```python
from build123d import *

# Parameters (mm, degrees)
SKETCH1_R               = 17.78
BOSS_EXTRUDE1_DEPTH     = 177.8
SKETCH9_R               = 23.495
BOSS_EXTRUDE4_DEPTH     = 12.7
MIRROR6_COPY_1_SKETCH_R = 23.495
MIRROR6_COPY_1_DEPTH    = 12.7
MIRROR6_COPY_2_SKETCH_R = 23.495
MIRROR6_COPY_2_DEPTH    = 12.7
MIRROR7_COPY_1_SKETCH_R = 23.495
MIRROR7_COPY_1_DEPTH    = 12.7
MIRROR7_COPY_2_SKETCH_R = 23.495
MIRROR7_COPY_2_DEPTH    = 12.7
MIRROR7_COPY_3_SKETCH_R = 23.495
MIRROR7_COPY_3_DEPTH    = 12.7
SKETCH13_R              = 88.9
BOSS_EXTRUDE6_DEPTH     = 76.2
FILLET3_R               = 25.4
FILLET4_R               = 25.4
FILLET3_OF_MIRROR11_R   = 25.4
FILLET4_OF_MIRROR11_R   = 25.4


with BuildPart() as part:
    # Sketch1 → Boss-Extrude1 (new, symmetric)
    with BuildSketch(Plane(origin=(0, 0, 0), x_dir=(0, 0, -1), z_dir=(1, 0, 0))):
        Circle(SKETCH1_R)
    extrude(amount=BOSS_EXTRUDE1_DEPTH, both=True)

    # Sketch9 → Boss-Extrude4 (add)
    with BuildSketch(Plane(origin=(177.8, 0, 0), x_dir=(0, 0, -1), z_dir=(1, 0, 0))):
        Circle(SKETCH9_R)
    boss_extrude4 = extrude(amount=BOSS_EXTRUDE4_DEPTH)

    # Mirror5: Boss-Extrude4 across plane
    add(boss_extrude4.mirror(Plane(origin=(0, 0, 0), x_dir=(0, 0, 1), z_dir=(1, 0, 0))))

    # Mirror6 copy 1 sketch → Mirror6 copy 1 (add)
    with BuildSketch(Plane.ZY.offset(177.8)):
        Circle(MIRROR6_COPY_1_SKETCH_R)
    extrude(amount=MIRROR6_COPY_1_DEPTH)

    # Mirror6 copy 2 sketch → Mirror6 copy 2 (add)
    with BuildSketch(Plane(origin=(177.8, 0, 0), x_dir=(0, 0, 1), z_dir=(1, 0, 0))):
        Circle(MIRROR6_COPY_2_SKETCH_R)
    extrude(amount=MIRROR6_COPY_2_DEPTH)

    # Mirror7 copy 1 sketch → Mirror7 copy 1 (add)
    with BuildSketch(Plane(origin=(-177.8, 0, 0), x_dir=(0, 0, -1), z_dir=(-1, 0, 0))):
        Circle(MIRROR7_COPY_1_SKETCH_R)
    extrude(amount=MIRROR7_COPY_1_DEPTH)

    # Mirror7 copy 2 sketch → Mirror7 copy 2 (add)
    with BuildSketch(Plane(origin=(177.8, 0, 0), x_dir=(0, 0, -1), z_dir=(1, 0, 0))):
        Circle(MIRROR7_COPY_2_SKETCH_R)
    extrude(amount=MIRROR7_COPY_2_DEPTH)

    # Mirror7 copy 3 sketch → Mirror7 copy 3 (add)
    with BuildSketch(Plane(origin=(177.8, 0, 0), x_dir=(0, 0, 1), z_dir=(1, 0, 0))):
        Circle(MIRROR7_COPY_3_SKETCH_R)
    extrude(amount=MIRROR7_COPY_3_DEPTH)

    # Sketch13 → Boss-Extrude6 (add)
    with BuildSketch(Plane(origin=(190.5, 0, 0), x_dir=(0, 0, -1), z_dir=(1, 0, 0))):
        with Locations(Location((0, 0, 0), (0, 0, 180))):
            Circle(SKETCH13_R)
    boss_extrude6 = extrude(amount=BOSS_EXTRUDE6_DEPTH)

    # Fillet3
    fillet3_edges = [part.edges().sort_by_distance(p)[0] for p in [
        (266.7, 0, -88.9),
    ]]
    fillet(fillet3_edges, radius=FILLET3_R)

    # Fillet4
    fillet4_edges = [part.edges().sort_by_distance(p)[0] for p in [
        (190.5, 0, -88.9),
    ]]
    fillet(fillet4_edges, radius=FILLET4_R)

    # Mirror11: Boss-Extrude6 across plane
    add(boss_extrude6.mirror(Plane(origin=(0, 0, 0), x_dir=(0, 0, 1), z_dir=(1, 0, 0))))

    # Fillet3 of Mirror11
    fillet3_of_mirror11_edges = [part.edges().sort_by_distance(p)[0] for p in [
        (-266.7, 0, -88.9),
    ]]
    fillet(fillet3_of_mirror11_edges, radius=FILLET3_OF_MIRROR11_R)

    # Fillet4 of Mirror11
    fillet4_of_mirror11_edges = [part.edges().sort_by_distance(p)[0] for p in [
        (-190.5, 0, -88.9),
    ]]
    fillet(fillet4_of_mirror11_edges, radius=FILLET4_OF_MIRROR11_R)


solid = part.part
```
The listing builds one solid part. Answer for the finished solid, in the listing's coordinates (mm). A direction names the side the tool comes from. Round coordinates to 2 decimals unless told otherwise and drop trailing zeros. Write each loop counter-clockwise with the first axis right and the second up, starting at its lowest first coordinate (ties: lowest second). Pieces come first, ordered by that corner, then holes. Notation, with made-up numbers: (-7, -32.5) -> (12, -32.5) arc R27 cw to (12, -9.5) -> close; hole circle Ø11 at (12.5, -37). An arc over 180 degrees is marked (long way). Answer as a JSON object with one key per item and string values. Group by question number.
Q1. Which of the six approach directions +Z, -Z, +X, -X, +Y, -Y give full straight-line access (tool end or side, diameter ignored) to faces 4 (the face through (177.8, 18, 4)), 5 (the face through (228.422, -60.083, -65.523))?
Q2. Each of these flat-tipped pins is pushed along its axis until it touches: pin 1 Ø12 at (y, z) = (0, -70.5) entering from +X; pin 2 Ø1 at (x, z) = (184, -1) entering from +Y; pin 3 Ø3 at (x, y) = (-75, 5) entering from +Z. Where does it stop, or does it pass through?
Q3. Straight lines are drawn through the part: line 1 along X through (y, z) = (53, -8.5); line 2 along X through (y, z) = (-7.5, 65); line 3 along Z through (x, y) = (31.5, -2). For each, find the intervals that lie inside material, in ascending order.
Q4. Determine the mould class of faces 1 (the face through (184.061, -22.936, 5.093)), 2 (the face through (-228.422, -60.083, -65.523)), 3 (the face through (-266.7, -1, -1)) for opening direction X: pulls with the +X half, pulls with the -X half, needs draft (parallel to the pull), parting line crosses it, or undercut.
Q5. Section A-A (y = 0) is taken. Write down the section's boundary in (x, z) (3 decimals).
Q6. Section D-D (x = -42) is taken. Write down the section's boundary in (y, z), plus the area to 3 significant figures.
Q7. Section C-C (x = -234) is taken. Write down the section's boundary in (y, z).
Check values:
{
 "1": {"face 4": "none", "face 5": "+X, -X"},
 "2": {"pin 1": "x = 266.68", "pin 2": "y = 23.49", "pin 3": "z = 17.43"},
 "3": {"line 1": "-266.7 to -190.5, 190.5 to 266.7", "line 2": "-266.63 to -190.57, 190.57 to 266.63", "line 3": "-17.67 to 17.67"},
 "4": {"face 1": "undercut", "face 2": "needs draft", "face 3": "pulls with the -X half"},
 "5": {"outline": "(-266.7, -63.5) arc R25.4 ccw to (-241.3, -88.9) -> (-215.9, -88.9) arc R25.4 ccw to (-190.5, -63.5) -> (-190.5, -23.495) -> (-177.8, -23.495) -> (-177.8, -17.78) -> (177.8, -17.78) -> (177.8, -23.495) -> (190.5, -23.495) -> (190.5, -63.5) arc R25.4 ccw to (215.9, -88.9) -> (241.3, -88.9) arc R25.4 ccw to (266.7, -63.5) -> (266.7, 63.5) arc R25.4 ccw to (241.3, 88.9) -> (215.9, 88.9) arc R25.4 ccw to (190.5, 63.5) -> (190.5, 23.495) -> (177.8, 23.495) -> (177.8, 17.78) -> (-177.8, 17.78) -> (-177.8, 23.495) -> (-190.5, 23.495) -> (-190.5, 63.5) arc R25.4 ccw to (-215.9, 88.9) -> (-241.3, 88.9) arc R25.4 ccw to (-266.7, 63.5) -> close"},
 "6": {"outline": "circle Ø35.56 at (0, 0)", "area": "993 mm^2"},
 "7": {"outline": "circle Ø177.8 at (0, 0)"}
}
